Autodesk Inventor part; units mm, degrees
ref_plane "YZ Plane" through (0, 0, 0) normal (1, 0, 0) x (0, 1, 0)
ref_plane "XZ Plane" through (0, 0, 0) normal (0, 1, 0) x (-1, 0, 0)
ref_plane "XY Plane" through (0, 0, 0) normal (0, 0, 1) x (1, 0, 0)
sketch "Sketch1" plane through (0, 0, 0) normal (0, 1, 0) x (-1, 0, 0)
  line L0 (14, 0) -> (-14, 0)
  line L1 (0, -48) -> (0, 8)
  line L2 (10, -40) -> (-10, -40)
  line L3 (-10, -40) -> (-10, 0)
  line L4 (-10, 0) -> (10, 0)
  line L5 (10, 0) -> (10, -40)
  point P0 (0, 0)
  dimension "d0" = 20
  dimension "d1" = 40
  dimension "d4" = 10
extrude "Extrusion1" add sketch "Sketch1" along normal blind 2
sketch "Sketch2" plane through (0, 2, 0) normal (0, 1, 0) x (1, 0, 0)
  line L0 (10, 40) -> (-10, 40)
  line L1 (-10, 40) -> (-10, 0)
  line L2 (-10, 0) -> (10, 0)
  line L3 (10, 0) -> (10, 40)
  line L4 (10, 13.5) -> (-10, 13.5) construction
  line L5 (-10, 13.5) -> (-10, 24.5) construction
  line L6 (-10, 24.5) -> (10, 24.5) construction
  line L7 (10, 24.5) -> (10, 13.5) construction
  line L8 (10, 0) -> (10, 40)
  arc A0 (4.5, 8) -> (7.5, 8) centre (6, 8) ccw
  arc A1 (-7.5, 8) -> (-4.5, 8) centre (-6, 8) ccw
  line L9 (0, 49.0401) -> (0, -8.1733) construction
  arc A2 (7.5, 9) -> (4.5, 9) centre (6, 9) ccw
  arc A3 (-4.5, 9) -> (-7.5, 9) centre (-6, 9) ccw
  line L10 (7.5, 8) -> (7.5, 9)
  line L11 (4.5, 8) -> (4.5, 9)
  line L12 (-4.5, 8) -> (-4.5, 9)
  line L13 (-7.5, 8) -> (-7.5, 9)
  circle A4 centre (-7, 27.5) radius 1
  line L14 (-7, 27.5) -> (15.2836, 27.5) construction
  line L15 (-7, 27.5) -> (11.3667, 45.8667) construction
  arc A5 (3.6066, 38.1066) -> (2.1834, 36.6834) centre (2.895, 37.395) ccw
  arc A6 (6, 27.5) -> (8, 27.5) centre (7, 27.5) ccw
  arc A7 (6, 27.5) -> (2.0828, 36.8006) centre (-7, 27.5) ccw
  arc A8 (8, 27.5) -> (3.6066, 38.1066) centre (-7, 27.5) ccw
  point P0 (0, 0)
  dimension "d6" = 11
  dimension "d8" = 3
  dimension "d9" = 3
  dimension "d10" = 8
  dimension "d11" = 8
  dimension "d12" = 6
  dimension "d13" = 6
  dimension "d14" = 3
  dimension "d15" = 3
  dimension "d16" = 4.5
  dimension "d17" = 2
  dimension "d18" = 3
  dimension "d19" = 3
  dimension "d22" = 45
extrude "Extrusion2" cut sketch "Sketch2" against normal blind 3 contours L11 A2 L10 A0 | L13 A3 L12 A1 | A4 | A8 A6 A7 A5
equation "\"d4\" = 0.5 * d0"
equation "\"d11\" = d10"
equation "\"d13\" = d12"
equation "\"d23\" = d15"
properties part number "BallBalancing_Hinge"
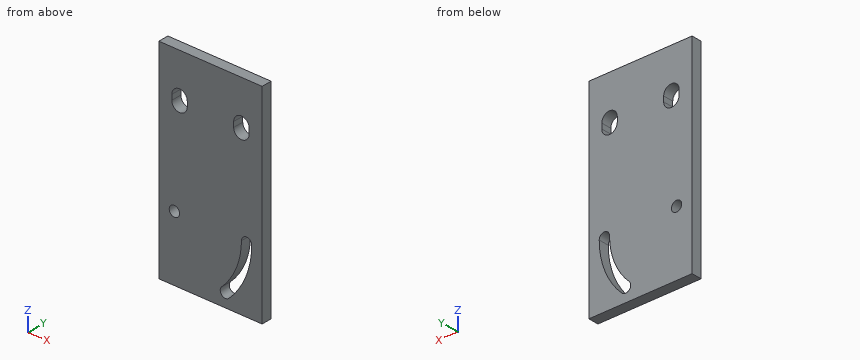
The listing builds one solid part. Answer for the finished solid, in the listing's coordinates (mm). Round coordinates to 2 decimals unless told otherwise and drop trailing zeros. Order: outer loops, then holes, each group sorted by start corner. A loop starts at its lowest first (then second) coordinate and runs counter-clockwise, first axis right, second up. Notation, with made-up numbers: (-20, 6) -> (34, 6) arc R23 ccw to (34, 14) -> close; hole circle Ø1 at (12.5, 55.25). An arc over 180 degrees is marked (long way). Put each result on its own line as item: value.
Q1. Section A-A, the plane x = -7 is taken. Write down the section's boundary in (y, z), and give its area (3 significant figures).
Results list:
outline: (0, -40) -> (2, -40) -> (2, -28.5) -> (0, -28.5) -> close; (0, -26.5) -> (2, -26.5) -> (2, -10.12) -> (0, -10.12) -> close; (0, -6.88) -> (2, -6.88) -> (2, 0) -> (0, 0) -> close
area: 69.5 mm^2
Q2. Section D-D, the plane x = 7 is taken. Write down the section's boundary in (y, z).
Results list:
outline: (0, -40) -> (2, -40) -> (2, -32.89) -> (0, -32.89) -> close; (0, -26.5) -> (2, -26.5) -> (2, -10.12) -> (0, -10.12) -> close; (0, -6.88) -> (2, -6.88) -> (2, 0) -> (0, 0) -> close
Q3. Section C-C, the plane y = 1 is taken. Write down the section's boundary in (x, z) (3 decimals).
Results list:
outline: (-10, -40) -> (10, -40) -> (10, 0) -> (-10, 0) -> close; hole circle Ø2 at (-7, -27.5); hole (-7.5, -9) arc R1.5 ccw to (-4.5, -9) -> (-4.5, -8) arc R1.5 ccw to (-7.5, -8) -> close; hole (2.083, -36.801) arc R1.006 ccw to (3.607, -38.107) arc R15 ccw to (8, -27.5) arc R1 ccw to (6, -27.5) arc R13 cw to start; hole (4.5, -9) arc R1.5 ccw to (7.5, -9) -> (7.5, -8) arc R1.5 ccw to (4.5, -8) -> close
Q4. Consider line 1 along X through (y, z) = (1, -9); line 2 along X through (y, z) = (1.55, -27.5); line 3 along Z through (x, y) = (-7, 0.8). Determine where each line is inside the solid, lowest interval first.
Results list:
line 1: -10 to -7.5, -4.5 to 4.5, 7.5 to 10
line 2: -10 to -8, -6 to 6, 8 to 10
line 3: -40 to -28.5, -26.5 to -10.12, -6.88 to 0
Q5. This flat-tipped pin is pushed along its axis until it touches: P1, Ø1, axis at x = 3, y = 1, coming from the +Z side. Where does it stop, or does it pass through?
Results list:
P1: z = 0
Q6. Section B-B, the plane z = -29 is taken. Write down the section's boundary in (x, y).
Results list:
outline: (-10, 0) -> (5.91, 0) -> (5.91, 2) -> (-10, 2) -> close; (7.92, 0) -> (10, 0) -> (10, 2) -> (7.92, 2) -> close
